Check sheet for the modelled part. Datum: model origin and axes. Units: mm. A direction names the side the tool comes from. Give positions to 0.01 mm unless a question says otherwise; leave off trailing zeros. Loops run counter-clockwise (first coordinate to the right, second up) from the corner with the lowest first, then second, coordinate; pieces in that order, holes last. Notation, with made-up numbers: (71.5, 46.25) -> (98.5, 46.25) arc R24 ccw to (98.5, 77.25) -> close; hole circle Ø4 at (1, 45.25). An arc over 180 degrees is marked (long way). Answer as CSV lines item,"result". Start each with the question number.
(1) Access from +Z, -Z, +X, -X, +Y, -Y to the whole of each face (thin tool, end or side, straight path). Record for faces 1 (the face through (1, -10, 3.5)), 2 (the face through (25.861, -0.229, 27.048)), 3 (the face through (25.861, -20.091, 27.048)).
(2) Material ranges on line 1 (Z direction, x = -32, y = -5.5); line 2 (Z direction, x = -30, y = -15.5); line 3 (X direction, y = -5, z = 8.5), recorded low to high. Write a range as from..to.
(3) Release check for a two-part mould opening along Z. For faces 4 (the face through (-36.4, -10, 7.5)), 5 (the face through (33.759, -10, 2)), 6 (the face through (31.92, -10.03, 30.17)), 7 (the face through (17.652, -10.028, 24.563)) record: pulls with the +Z half, pulls with the -Z half, needs draft (parallel to the pull), parting line crosses it, or undercut.
(4) Section check A-A on y = -5. Enter the section's corners in (x, z).
(5) Gauge pin test, flat ends, axial feed: pin 1 Ø1.5 at (x, y) = (1.5, -3) entering from +Z; pin 2 Ø12 at (y, z) = (-17, 26.5) entering from +X; pin 3 Ø1 at (x, y) = (-13.5, -15) entering from +Z. Record the tip position at first contact, or that the pin passes through.
from build123d import *

# Parameters (mm, degrees)
F1_DEPTH = 20.32
F2_R     = 0.762


with BuildPart() as f1:
    # F0 (on Front) → F1 (new body)
    with BuildSketch(Plane.XZ):
        with BuildLine():
            Line((-32.2812777423, 0), (33.7587222577, 0))
            Line((33.7587222577, 0), (33.7587222577, 3.5))
            Line((33.7587222577, 3.5), (-32.2812777423, 3.5))
            ThreePointArc((-32.2812777423, 3.5), (-36.4012550506, 7.6063259449), (-32.308625702, 11.7399092331))
            ThreePointArc((-32.308625702, 11.7399092331), (-7.7452704082, 14.8185162016), (15.4165966965, 23.5571749303))
            ThreePointArc((15.4165966965, 23.5571749303), (17.6844448263, 24.575463703), (20.0530860269, 25.3301729364))
            Line((20.0530860269, 25.3301729364), (32.3530167072, 28.49272021))
            Line((32.3530167072, 28.49272021), (31.481448561, 31.8824648857))
            Line((31.481448561, 31.8824648857), (19.1815178806, 28.7199176121))
            ThreePointArc((19.1815178806, 28.7199176121), (16.4343267164, 27.8445927478), (13.8040371048, 26.6635637603))
            ThreePointArc((13.8040371048, 26.6635637603), (-8.5865023609, 18.215916502), (-32.331858192, 15.2398321253))
            ThreePointArc((-32.331858192, 15.2398321253), (-39.9012357736, 7.5947096359), (-32.2812777423, 0))
        make_face()
    extrude(amount=F1_DEPTH)

    # F2
    f2_edges = [f1.edges().sort_by_distance(p)[0] for p in [
        (16.434327, -20.32, 27.844593),
        (-8.586502, -20.32, 18.215917),
        (-39.901236, -20.32, 7.59471),
        (0.738722, -20.32, 0),
        (33.758722, -20.32, 1.75),
        (0.738722, -20.32, 3.5),
        (-36.401255, -20.32, 7.606326),
        (-7.74527, -20.32, 14.818516),
        (17.684445, -20.32, 24.575464),
        (26.203051, -20.32, 26.911447),
        (31.917233, -20.32, 30.187593),
        (25.331483, -20.32, 30.301191),
        (16.434327, 0, 27.844593),
        (-8.586502, 0, 18.215917),
        (-39.901236, 0, 7.59471),
        (0.738722, 0, 0),
        (33.758722, 0, 1.75),
        (0.738722, 0, 3.5),
        (-36.401255, 0, 7.606326),
        (-7.74527, 0, 14.818516),
        (17.684445, 0, 24.575464),
        (26.203051, 0, 26.911447),
        (31.917233, 0, 30.187593),
        (25.331483, 0, 30.301191),
        (32.353017, -10.16, 28.49272),
        (31.481449, -10.16, 31.882465),
        (33.758722, -10.16, 0),
        (33.758722, -10.16, 3.5),
    ]]
    fillet(f2_edges, radius=F2_R)


solid = f1.part
Working result:
1,face 1,"+X, +Y, -Y"
1,face 2,"+X, +Y"
1,face 3,"+X, -Y"
2,line 1,"z = 0..3.5, 11.74..15.24"
2,line 2,"z = 0..3.5, 11.78..15.28"
2,line 3,"x = -39.85..-36.31"
3,face 4,"undercut"
3,face 5,"needs draft"
3,face 6,"pulls with the +Z half"
3,face 7,"undercut"
4,outline,"(-32.33, 15.24) arc R7.62 ccw to (-32.28, 0) -> (33, 0) arc R0.76 ccw to (33.76, 0.76) -> (33.76, 2.74) arc R0.76 ccw to (33, 3.5) -> (-32.28, 3.5) arc R4.12 cw to (-32.31, 11.74) arc R105.1 ccw to (15.42, 23.56) arc R21.9 cw to (20.05, 25.33) -> (31.62, 28.3) arc R0.76 ccw to (32.16, 29.23) -> (31.67, 31.14) arc R0.76 ccw to (30.74, 31.69) -> (19.18, 28.72) arc R25.4 ccw to (13.8, 26.66) arc R101.6 cw to start"
5,pin 1,"stops at z = 21.55"
5,pin 2,"stops at x = 32.19"
5,pin 3,"stops at z = 17.23"
